from build123d import *

# Parameters (mm, degrees)
EXTRUDE_THIN1_DEPTH = 200
CUT_EXTRUDE1_DEPTH  = 1
LPATTERN1_COUNT     = 9
LPATTERN1_PITCH     = 25


with BuildPart() as part:
    # Sketch1 → Extrude-Thin1 (new body)
    with BuildSketch(Plane(origin=(0, 0, 0), x_dir=(0, 0, -1), z_dir=(1, 0, 0))):
        with BuildLine():
            Line((-17.5, 6.5), (-15.5, 6.5))
            ThreePointArc((-15.5, 6.5), (-14.085786438, 5.914213562), (-13.5, 4.5))
            Line((-13.5, 4.5), (-13.5, 2))
            ThreePointArc((-13.5, 2), (-12.914213562, 0.585786438), (-11.5, 0))
            Line((-11.5, 0), (11.5, 0))
            ThreePointArc((11.5, 0), (12.914213562, 0.585786438), (13.5, 2))
            Line((13.5, 2), (13.5, 4.5))
            ThreePointArc((13.5, 4.5), (14.085786438, 5.914213562), (15.5, 6.5))
            Line((15.5, 6.5), (17.5, 6.5))
            Line((17.5, 6.5), (17.5, 7.5))
            Line((17.5, 7.5), (15.5, 7.5))
            ThreePointArc((15.5, 7.5), (13.378679656, 6.621320344), (12.5, 4.5))
            Line((12.5, 4.5), (12.5, 2))
            ThreePointArc((12.5, 2), (12.207106781, 1.292893219), (11.5, 1))
            Line((11.5, 1), (-11.5, 1))
            ThreePointArc((-11.5, 1), (-12.207106781, 1.292893219), (-12.5, 2))
            Line((-12.5, 2), (-12.5, 4.5))
            ThreePointArc((-12.5, 4.5), (-13.378679656, 6.621320344), (-15.5, 7.5))
            Line((-15.5, 7.5), (-17.5, 7.5))
            Line((-17.5, 7.5), (-17.5, 6.5))
        make_face()
    extrude(amount=EXTRUDE_THIN1_DEPTH)

    # Sketch2 → Cut-Extrude1 (cut)
    with BuildSketch(Plane.XZ):
        with BuildLine():
            Line((-5.875, 3.125), (5.875, 3.125))
            ThreePointArc((5.875, 3.125), (9, 0), (5.875, -3.125))
            Line((5.875, -3.125), (-5.875, -3.125))
            ThreePointArc((-5.875, -3.125), (-9, 0), (-5.875, 3.125))
        make_face()
    cut_extrude1 = extrude(amount=-CUT_EXTRUDE1_DEPTH, mode=Mode.SUBTRACT)

    # LPattern1: Cut-Extrude1 ×9
    with Locations(*[(i * LPATTERN1_PITCH, 0, 0) for i in range(1, LPATTERN1_COUNT)]):
        add(cut_extrude1, mode=Mode.SUBTRACT)


solid = part.part
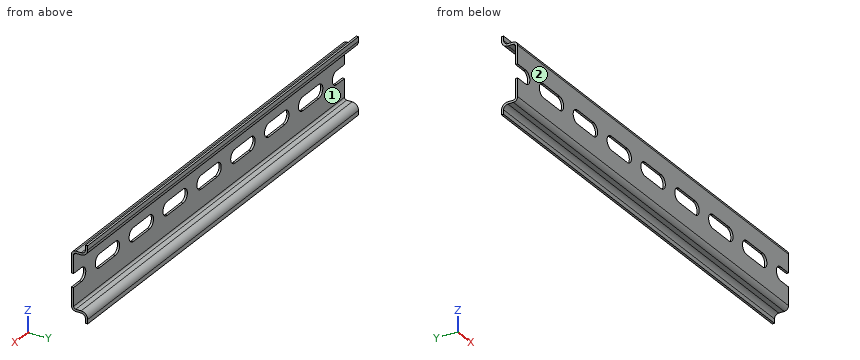
Build history of the part. All positions in model axes, mm. Face numbers are marked on the shaded views. Coordinates: 2 decimals unless noted, no trailing zeros. Write item = value, one per line. Start each with the question number.
1) Wall check: line 1 along Z through (x, y) = (151.5, 2.5); line 2 along Y through (x, z) = (175, 6); line 3 along Z through (x, y) = (115, 6.75). Give the ranges that are in metal, low to high. Write a range as from..to.
2) Flat gauge pins, fed straight in: pin 1 Ø0.8 at (x, y) = (151, 0.5) entering from -Z; pin 2 Ø1.1 at (x, y) = (197, 0.5) entering from +Z; pin 3 Ø2 at (x, y) = (68, 3) entering from -Z; pin 4 Ø1 at (y, z) = (2.5, -3) entering from -X. Where does each tip first touch, or does it go through?
3) Saw through at A-A on z = 0. Count the separate pieces of the cut face and the enclosed holes in it, then the cut area to 3 significant figures.
4) Two-plate mould, pull along Z, no slides. Class the marked faces 1 and 2: pulls with the +Z half, pulls with the -Z half, needs draft (parallel to the pull), parting line crosses it, or undercut.
From the geometry:
q1.line_1 = -13.5..-12.5, 12.5..13.5
q1.line_2 = 0..1
q1.line_3 = -17.5..-13.52, 13.52..17.5
q2.pin_1 = -13.17
q2.pin_2 = 13.26
q2.pin_3 = -13.5
q2.pin_4 = through
q3.separate_pieces = 8
q3.enclosed_holes = 0
q3.area = 56.0 mm^2
q4.face_1 = undercut
q4.face_2 = needs draft
